from build123d import *

# Parameters (mm, degrees)
SKETCH1_R           = 17.78
BOSS_EXTRUDE1_DEPTH = 33.02
SKETCH2_R           = 18.415
BOSS_EXTRUDE2_DEPTH = 23.1775
SKETCH3_R           = 1.524
CUT_EXTRUDE1_DEPTH  = 12.7
SKETCH4_R           = 5.969
BOSS_EXTRUDE3_DEPTH = 4.826
BOSS_EXTRUDE4_DEPTH = 14.732


with BuildPart() as part:
    # Sketch1 → Boss-Extrude1 (new body)
    with BuildSketch(Plane(origin=(0, 0, 0), x_dir=(1, 0, 0), z_dir=(0, 1, 0))):
        Circle(SKETCH1_R)
    extrude(amount=BOSS_EXTRUDE1_DEPTH)

    # Sketch2 → Boss-Extrude2 (add)
    with BuildSketch(Plane(origin=(0, 33.02, 0), x_dir=(1, 0, 0), z_dir=(0, 1, 0))):
        Circle(SKETCH2_R)
    extrude(amount=BOSS_EXTRUDE2_DEPTH)

    # Sketch3 → Cut-Extrude1 (cut)
    with BuildSketch(Plane(origin=(0, 56.1975, 0), x_dir=(1, 0, 0), z_dir=(0, 1, 0))):
        with Locations((15.24, 0)):
            Circle(SKETCH3_R)
        with Locations((7.62, -13.198227154)):
            Circle(SKETCH3_R)
        with Locations((-7.62, -13.198227154)):
            Circle(SKETCH3_R)
        with Locations((-15.24, 0)):
            Circle(SKETCH3_R)
        with Locations((-7.62, 13.198227154)):
            Circle(SKETCH3_R)
        with Locations((7.62, 13.198227154)):
            Circle(SKETCH3_R)
    extrude(amount=-CUT_EXTRUDE1_DEPTH, mode=Mode.SUBTRACT)

    # Sketch4 → Boss-Extrude3 (add)
    with BuildSketch(Plane(origin=(0, 56.1975, 0), x_dir=(1, 0, 0), z_dir=(0, 1, 0))):
        with Locations((0, -6.985)):
            Circle(SKETCH4_R)
    extrude(amount=BOSS_EXTRUDE3_DEPTH)

    # Sketch5 → Boss-Extrude4 (add)
    with BuildSketch(Plane(origin=(0, 61.0235, 0), x_dir=(1, 0, 0), z_dir=(0, 1, 0))):
        with BuildLine():
            Line((1.665589385, -9.4615), (-1.665589385, -9.4615))
            ThreePointArc((-1.665589385, -9.4615), (0, -4.0005), (1.665589385, -9.4615))
        make_face()
    extrude(amount=BOSS_EXTRUDE4_DEPTH)


solid = part.part
Design review of the part built by this model. Coordinates are the model's own, in mm. A direction names the side the tool comes from. Round coordinates to 2 decimals unless told otherwise and drop trailing zeros. Order: outer loops, then holes, each group sorted by start corner. A loop starts at its lowest first (then second) coordinate and runs counter-clockwise, first axis right, second up. Notation, with made-up numbers: M 75.25,-23 L 122.25,-23 A27 ccw 122.25,-3 Z; hole C 76,88 d11. An arc over 180 degrees is marked long. Answer as CSV lines item,"result". Start each with the question number.
1) Add section B-B (z = 0). Give the boundary of the cut face in (x, y) (1 decimal).
2) Tool access review of faces 1 (the face through (-8, 43.498, 13)), 2 (the face through (-3.85, 16.28, 17.36)), 3 (the face through (0, 68, 9.462)): name each direction out of +Z, -Z, +X, -X, +Y, -Y from which nothing blocks a thin tool from reaching the whole face with its end or side.
3) The part is to be moulded in two halves that separate along Z. For faces 4 (the face through (0, 61.024, 10)), 5 (the face through (-0.777, 58.577, 1.067)), 6 (the face through (8, 43.498, -13)), 7 (the face through (-15, 43.498, 0)), say which applies: +Z half, -Z half, draft (parallel to the pull), parting line (faces both ways), or undercut.
4) For pin 1 Ø2.5 at (x, z) = (-8, 14) entering from +Y; pin 2 Ø12 at (y, z) = (11, -7.5) entering from -X; pin 3 Ø0.9 at (x, z) = (-14.5, -0.5) entering from +Y, all flat-tipped, find the tip position at first contact; note any pin that passes through.
5) Wall thickness on line 1 along X through (y, z) = (49, 0) (3 decimals); line 2 along Z through (x, y) = (-7.62, 49.25); line 3 along Y through (x, z) = (-7, -1): over which ranges is each line inside the solid? List them lowest first. Write a range as [from, to].
6) Add section A-A (x = 0). Give the boundary of the cut face in (y, z) (1 decimal).
7) Add section D-D (y = 41). Give the boundary of the cut face in (x, z) (3 decimals).
8) Add section C-C (y = 50.5). Give the boundary of the cut face in (x, z) (3 decimals).
Resolved:
1,outline,"M -18.4,33 L -17.8,33 L -17.8,0 L 17.8,0 L 17.8,33 L 18.4,33 L 18.4,56.2 L 16.8,56.2 L 16.8,43.5 L 13.7,43.5 L 13.7,56.2 L -13.7,56.2 L -13.7,43.5 L -16.8,43.5 L -16.8,56.2 L -18.4,56.2 Z"
2,face 1,"+Y"
2,face 2,"-Y"
2,face 3,"+Z, +X, -X, +Y"
3,face 4,"draft"
3,face 5,"parting line"
3,face 6,"undercut"
3,face 7,"undercut"
4,pin 1,"y = 56.2"
4,pin 2,"x = -17.72"
4,pin 3,"y = 43.5"
5,line 1,"[-18.415, -16.764], [-13.716, 13.716], [16.764, 18.415]"
5,line 2,"[-16.76, -14.72], [-11.67, 11.67], [14.72, 16.76]"
5,line 3,"[0, 56.2]"
6,outline,"M 0,-17.8 L 33,-17.8 L 33,-18.4 L 56.2,-18.4 L 56.2,1 L 61,1 L 61,4 L 75.8,4 L 75.8,9.5 L 61,9.5 L 61,13 L 56.2,13 L 56.2,18.4 L 33,18.4 L 33,17.8 L 0,17.8 Z"
7,outline,"C 0,0 d36.83"
8,outline,"C 0,0 d36.83; hole C -15.24,0 d3.048; hole C -7.62,-13.198 d3.048; hole C -7.62,13.198 d3.048; hole C 7.62,-13.198 d3.048; hole C 7.62,13.198 d3.048; hole C 15.24,0 d3.048"
